Source: three-view drawing plus pictorial views. Frame: mm from the lowest corner of the part. Coordinates: 2 decimals unless noted, no trailing zeros. Order: outer loops, then holes, each group sorted by start corner. A loop starts at its lowest first (then second) coordinate and runs counter-clockwise, first axis right, second up. Notation, with made-up numbers: (3.5, 68.25) -> (59.5, 68.25) arc R15 ccw to (59.5, 81.25) -> close; hole circle Ø4 at (34.25, 13). An arc over 180 degrees is marked (long way). Use one line per item in the form item = value. Start each with the question number.
1) Pin query (flat end, axial travel): pin 1 (1 mm diameter, centred on x = 13, z = 6, fed in from -Y). Return the tip coordinate at first contact, or that it passes through.
2) Draft query along Z for the marked faces 1, 2 and 3. Return one class per face: pulls with the +Z half, pulls with the -Z half, needs draft (parallel to the pull), parting line crosses it, or undercut.
3) Section query A-A on y = 10. Output: boundary loops of the cut face in (x, z), then the cut area to 3 significant figures.
4) Ray query, line 1 along Y through (x, z) = (10, 1.75); line 2 along Z through (x, y) = (17.5, 16.5); line 3 along Y through (x, z) = (8.5, 5.25). Return the intervals inside material, ascending.
5) Section query D-D on x = 3.25. Output: boundary loops of the cut face in (y, z).
6) Section query C-C on z = 3. Output: boundary loops of the cut face in (x, y), then the cut area to 3 significant figures.
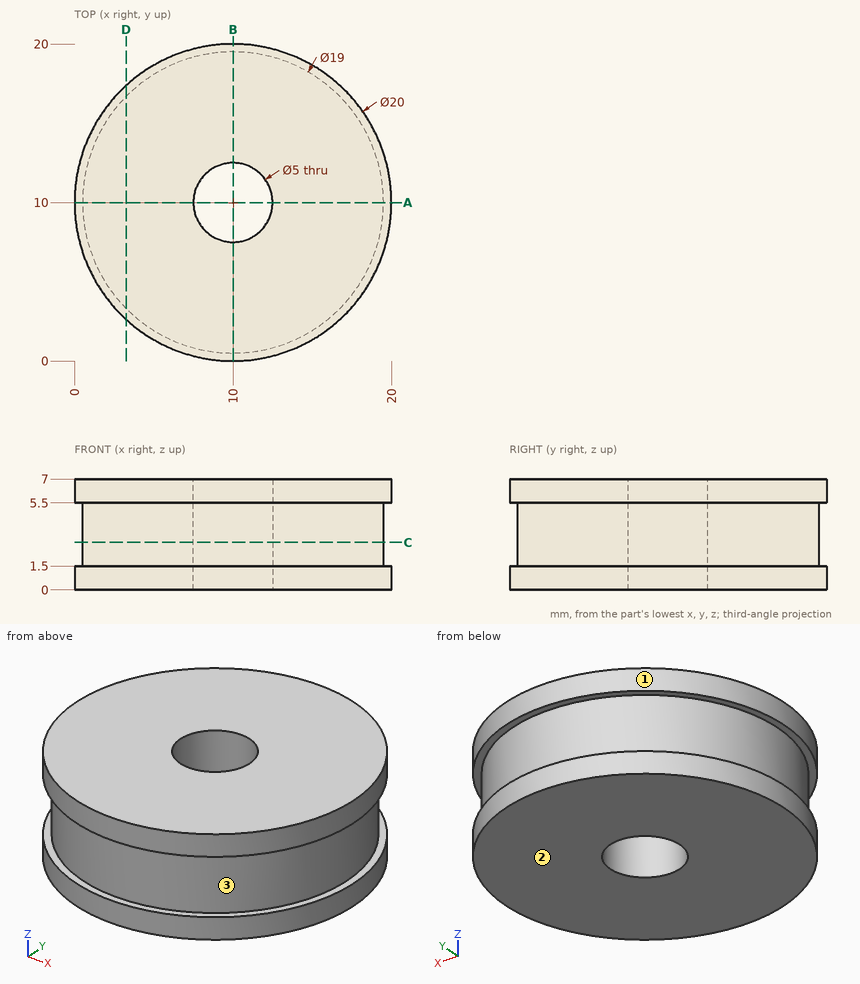
Answers below:
q1.pin_1 = 0.32
q2.face_1 = needs draft
q2.face_2 = pulls with the -Z half
q2.face_3 = undercut
q3.outline = (0, 0) -> (7.5, 0) -> (7.5, 7) -> (0, 7) -> (0, 5.5) -> (0.5, 5.5) -> (0.5, 1.5) -> (0, 1.5) -> close; (12.5, 0) -> (20, 0) -> (20, 1.5) -> (19.5, 1.5) -> (19.5, 5.5) -> (20, 5.5) -> (20, 7) -> (12.5, 7) -> close
q3.area = 101 mm^2
q4.line_1 = 0.5 to 7.5, 12.5 to 19.5
q4.line_2 = 0 to 1.5, 5.5 to 7
q4.line_3 = 0.62 to 8, 12 to 19.38
q5.outline = (2.62, 0) -> (17.38, 0) -> (17.38, 1.5) -> (16.68, 1.5) -> (16.68, 5.5) -> (17.38, 5.5) -> (17.38, 7) -> (2.62, 7) -> (2.62, 5.5) -> (3.32, 5.5) -> (3.32, 1.5) -> (2.62, 1.5) -> close
q6.outline = circle Ø19 at (10, 10); hole circle Ø5 at (10, 10)
q6.area = 264 mm^2
